```python
from build123d import *

# Parameters (mm, degrees)
EXTRUDE_1_DEPTH  = 6
MM_CLEARANCE_1_D = 3


with BuildPart() as part:
    # 草图1 → 凸台-拉伸1 (new body)
    with BuildSketch(Plane(origin=(0, 0, 0), x_dir=(0, 0, -1), z_dir=(1, 0, 0))):
        Polygon((0, 0), (0, 8), (4, 8), (4, 3.6), (17.3, 3.6), (17.3, 8), (21.3, 8), (21.3, 0), align=None)
    extrude(amount=EXTRUDE_1_DEPTH)

    # 大小mm Clearance 暗销孔1 (through all)
    with Locations(Plane(origin=(3, 8, -2), x_dir=(0, 0, 1), z_dir=(0, 1, 0))):
        with Locations((0, 0), (-17.3, 0)):
            Hole(MM_CLEARANCE_1_D / 2)


solid = part.part
```
CAD build for the part. Positions are in the model's coordinates, mm. A direction names the side the tool comes from. Give positions to 0.01 mm unless a question says otherwise; leave off trailing zeros. Order: outer loops, then holes, each group sorted by start corner. A loop starts at its lowest first (then second) coordinate and runs counter-clockwise, first axis right, second up.
(1) Tool access for faces 4 (the flat face through (3, 3.6, -11)), 5 (the cylindrical face through (2.1, 3.9, -0.8)): list every direction of +Z, -Z, +X, -X, +Y, -Y with a clear straight run to the whole face (end or side of a thin tool).
(2) Saw through at C-C, the plane x = 3. Give the cut face in (y, z), then the cut area to 3 significant figures.
(3) Saw through at B-B, the plane y = 4.75. Give the cut face in (x, z).
(4) Saw through at A-A, the plane z = -2. Give the cut face in (x, y).
(5) Mould opens along Z. For faces 1 (the flat face through (3, 4, 0)), 2 (the flat face through (1.6, 8, -1.1)), 3 (the flat face through (3, 6, -4)) say: released by +Z, released by -Z, zero draft, split by the parting line, or undercut.
(6) Saw through at D-D, the plane y = 2. Give the cut face in (x, z), then the cut area to 3 significant figures.
(7) Drill centre lines: L1, parallel to X at y = 6, z = -2; L2, parallel to Z at x = 2.05, y = 7.75; L3, parallel to Z at x = 3.3, y = 6.25. Where is each one in solid material? Low to high.
(8) Flat gauge pin, fed straight in: pin 1 (2 mm diameter, centred on x = 1, z = -7.5, fed in from +Y). Where does the tip first touch, or does it go through?
Results found:
1. face 4: +X, -X, +Y
1. face 5: +Y, -Y
2. outline: (0, -21.3) - (8, -21.3) - (8, -20.8) - (0, -20.8) - close; (0, -17.8) - (8, -17.8) - (8, -17.3) - (3.6, -17.3) - (3.6, -4) - (8, -4) - (8, -3.5) - (0, -3.5) - close; (0, -0.5) - (8, -0.5) - (8, 0) - (0, 0) - close
2. area: 63.9 mm2
3. outline: (0, -21.3) - (6, -21.3) - (6, -17.3) - (0, -17.3) - close; (0, -4) - (6, -4) - (6, 0) - (0, 0) - close; hole circle Ø3 at (3, -19.3); hole circle Ø3 at (3, -2)
4. outline: (0, 0) - (1.5, 0) - (1.5, 8) - (0, 8) - close; (4.5, 0) - (6, 0) - (6, 8) - (4.5, 8) - close
5. face 1: released by +Z
5. face 2: zero draft
5. face 3: undercut
6. outline: (0, -21.3) - (6, -21.3) - (6, 0) - (0, 0) - close; hole circle Ø3 at (3, -19.3); hole circle Ø3 at (3, -2)
6. area: 114 mm2
7. L1: x = 0 to 1.5, 4.5 to 6
7. L2: z = -21.3 to -20.46, -18.14 to -17.3, -4 to -3.16, -0.84 to 0
7. L3: z = -21.3 to -20.77, -17.83 to -17.3, -4 to -3.47, -0.53 to 0
8. pin 1: stops at y = 3.6
